Here's how the part is built. I have some questions about the finished solid (model axes, mm). Face numbers are marked on the shaded views. A direction names the side the tool comes from. Coordinates: 2 decimals unless noted, no trailing zeros. Loops run counter-clockwise (first coordinate to the right, second up) from the corner with the lowest first, then second, coordinate; pieces in that order, holes last.
from build123d import *

# Parameters (mm, degrees)
F0_R     = 3
F1_DEPTH = 7
F3_DEPTH = 2.5


with BuildPart() as f1:
    # F0 (on Right) → F1 (new body)
    with BuildSketch(Plane.YZ):
        Polygon((4.907477, 8.5), (-4.907477, 8.5), (-9.814955, 0), (-4.907477, -8.5), (4.907477, -8.5), (9.814955, 0), align=None)
        Circle(F0_R, mode=Mode.SUBTRACT)
    extrude(amount=F1_DEPTH)

    # F2 (on face) → F3 (cut)
    with BuildSketch(Plane(origin=(0, 0, 0), x_dir=(0, -1, 0), z_dir=(-1, 0, 0))):
        with BuildLine():
            Line((6, 1.3), (-6, 1.3))
            ThreePointArc((-6, 1.3), (-7.3, 0), (-6, -1.3))
            Line((-6, -1.3), (6, -1.3))
            ThreePointArc((6, -1.3), (7.3, 0), (6, 1.3))
        make_face()
    extrude(amount=-F3_DEPTH, mode=Mode.SUBTRACT)


solid = f1.part
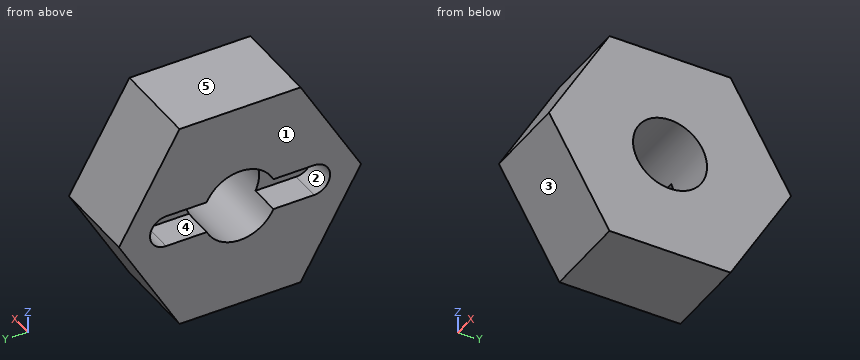
Q1. For the marked faces 1 and 2, which set-ups out of +Z, -Z, +X, -X, +Y, -Y let a thin tool reach every point of the face, with its end or its side?
Q2. We'd pull the mould along Y, two halves only. Please class the marked faces 3, 4 and 5: pulls with the +Y half, pulls with the -Y half, needs draft (parallel to the pull), parting line crosses it, or undercut.
Q3. Suppose I cut it at A-A on y = 0. Write out the boundary of the cut face in (x, z), and give its area (3 significant figures).
Q4. Suppose I cut it at B-B on x = 3.5. Write out the boundary of the cut face in (y, z), and give its area (3 significant figures).
Q5. Suppose I cut it at C-C on z = -2.25. Write out the boundary of the cut face in (x, y).
Q6. Will these pins go through, and if not, where does the flat tip stop? P1, Ø0.8, axis at y = -6, z = 0.5, coming from the -X side; P2, Ø2, axis at x = 5.5, z = -5, coming from the -Y side.
Q7. Please list where these lines run through material, in increasing order: probe 1 along Z at (x, y) = (4, 0); probe 2 along Z at (x, y) = (0.5, 4.5); probe 3 along Y at (x, z) = (5, -2.5).
Q8. Suppose I cut it at D-D on y = 3.5. Write out the boundary of the cut face in (x, z).
Check values:
1. face 1: +Z, -Z, -X, +Y, -Y
1. face 2: -X
2. face 3: pulls with the -Y half
2. face 4: undercut
2. face 5: needs draft
3. outline: (0, -8.5) - (7, -8.5) - (7, -3) - (0, -3) - close; (0, 3) - (7, 3) - (7, 8.5) - (0, 8.5) - close
3. area: 77.0 mm2
4. outline: (-9.81, 0) - (-4.91, -8.5) - (4.91, -8.5) - (9.81, 0) - (4.91, 8.5) - (-4.91, 8.5) - close; hole circle Ø6 at (0, 0)
4. area: 222 mm2
5. outline: (0, -8.52) - (7, -8.52) - (7, -1.98) - (0, -1.98) - close; (0, 1.98) - (7, 1.98) - (7, 8.52) - (0, 8.52) - close
6. P1: stops at x = 2.5
6. P2: stops at y = -7.51
7. probe 1: z = -8.5 to -3, 3 to 8.5
7. probe 2: z = -8.5 to -1.3, 1.3 to 8.5
7. probe 3: y = -8.37 to -1.66, 1.66 to 8.37
8. outline: (0, -8.5) - (7, -8.5) - (7, 8.5) - (0, 8.5) - (0, 1.3) - (2.5, 1.3) - (2.5, -1.3) - (0, -1.3) - close
